Read the model definition and answer for the solid it produces. Units are mm, in the model's axes. Face numbers are marked on the shaded views. Coordinates: 2 decimals unless noted, no trailing zeros. Write each loop counter-clockwise with the first axis right and the second up, starting at its lowest first coordinate (ties: lowest second). Pieces come first, ordered by that corner, then holes.
(1) Straight lines are drawn through the part: line 1 along X through (y, z) = (0, 2.25) (3 decimals); line 2 along Y through (x, z) = (1.25, -0.25); line 3 along Z through (x, y) = (0.75, 2.5). For each, find the intervals that lie inside material, in ascending order.
(2) Determine the mould class of the marked faces 1 and 2 for opening direction Y: pulls with the +Y half, pulls with the -Y half, needs draft (parallel to the pull), parting line crosses it, or undercut.
(3) The part is cut by section A-A, the plane z = -3.75. Determine the outline of the cut face in (x, y) (3 decimals).
(4) Given pin 1 (4 mm diameter, centred on y = -2, z = -2, fed in from +X) (3 decimals); pin 2 (1 mm diameter, centred on x = 1, y = 0, fed in from +Z) (3 decimals); pin 3 (1.5 mm diameter, centred on y = -2, z = 0.5, fed in from -X), each flat-ended and moving along its own axis, determine where each tip first touches the part or whether it passes through.
(5) The part is cut by section B-B, the plane z = 1.25. Determine the outline of the cut face in (x, y) (3 decimals), and give its area (3 significant figures).
Autodesk Inventor part; units mm, degrees
ref_plane "YZ Plane" through (0, 0, 0) normal (1, 0, 0) x (0, 1, 0)
ref_plane "XZ Plane" through (0, 0, 0) normal (0, 1, 0) x (-1, 0, 0)
ref_plane "XY Plane" through (0, 0, 0) normal (0, 0, 1) x (1, 0, 0)
sketch "Sketch1" plane through (0, 0, 0) normal (1, 0, 0) x (0, 1, 0)
  line L0 (0, 4.625) -> (0, -4.625)
  line L1 (0, -4.625) -> (1.625, -4.625)
  line L2 (1.625, -4.625) -> (1.625, 3.7361)
  arc A0 (1.8594, 4.1597) -> (3.5, 7.125) centre (0, 7.125) ccw
  arc A1 (0, 4.625) -> (2.5, 7.125) centre (0, 7.125) ccw
  line L3 (2.5, 7.125) -> (3.5, 7.125)
  arc A2 (1.8594, 4.1597) -> (1.625, 3.7361) centre (2.125, 3.7361) ccw
  point P0 (0, 0)
  point P1 (1.625, 4.0251)
  dimension "d0" = 11.75
  dimension "d1" = 1.625
  dimension "d2" = 2.5
  dimension "d3" = 3.5
  dimension "d4" = 0.5
revolve "Revolution1" add sketch "Sketch1" angle 360 about axis through (0, 0, 4.625) along (0, 0, -1)
sketch "Sketch2" plane through (0, 0, -4.625) normal (0, 0, -1) x (-1, 0, 0)
  circle A0 centre (0, 0) radius 1.625
  line L0 (0.5774, 1) -> (1.1547, 0)
  line L1 (1.1547, 0) -> (0.5774, -1)
  line L2 (0.5774, -1) -> (-0.5774, -1)
  line L3 (-0.5774, -1) -> (-1.1547, 0)
  line L4 (-1.1547, 0) -> (-0.5774, 1)
  line L5 (-0.5774, 1) -> (0.5774, 1)
  point P0 (0, 0)
  dimension "d6" = 2
extrude "Extrusion1" cut sketch "Sketch2" against normal blind 1.5 contours L0 L1 L2 L3 L4 L5
fillet "Fillet1" radius 0.2 1 edges at (0, -1.625, -4.625)
fillet "Fillet2" radius 0.5 2 edges at (0, -3.5, 7.125) (0, -2.5, 7.125)
thread "Thread2"
properties part number "Component 28 (Rocker Arm Linkage)"
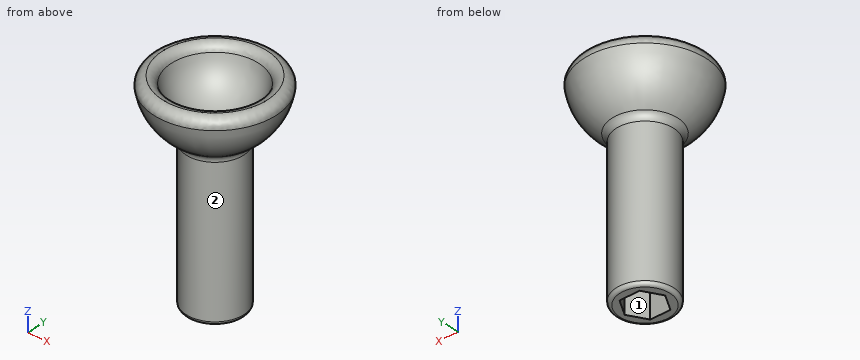
Computed:
1. line 1: x = -1.625 to 1.625
1. line 2: y = -1.04 to 1.04
1. line 3: z = 4.79 to 6.98
2. face 1: undercut
2. face 2: parting line crosses it
3. outline: circle Ø3.25 at (0, 0); hole (-1.155, 0) - (-0.577, -1) - (0.577, -1) - (1.155, 0) - (0.577, 1) - (-0.577, 1) - close
4. pin 1: stops at x = 1.625
4. pin 2: stops at z = 5.125
4. pin 3: stops at x = -1.04
5. outline: circle Ø3.25 at (0, 0)
5. area: 8.30 mm2
